```python
from build123d import *

# Parameters (mm, degrees)
PAD_DEPTH       = 20
SKETCH001_R     = 4.5
POCKET_DEPTH    = 107.001
SKETCH002_R     = 8.25
POCKET001_DEPTH = 25
POCKET002_DEPTH = 10
SKETCH004_R     = 1.5
POCKET003_DEPTH = 10.001
SKETCH005_R     = 5.5
POCKET004_DEPTH = 10
SKETCH006_W     = 23
SKETCH006_H     = 12
POCKET005_DEPTH = 3
SKETCH007_R     = 1.5
POCKET006_DEPTH = 7.001


with BuildPart() as part:
    # Sketch → Pad (new body)
    with BuildSketch(Plane.XY):
        with BuildLine():
            ThreePointArc((0, 57.5), (-57.5, 0), (0, -57.5))
            Line((0, -57.5), (0, -93.245553))
            Line((0, -93.245553), (-30, -93.245553))
            Line((-30, -93.245553), (-30, -63.245553))
            ThreePointArc((-55.235858, -43), (-43.803635, -54.600747), (-30, -63.245553))
            Line((-107, -20), (-55.235858, -43))
            Line((-107, 20), (-107, -20))
            Line((-55.235858, 43), (-107, 20))
            ThreePointArc((-30, 63.245553), (-43.803635, 54.600747), (-55.235858, 43))
            Line((-30, 93.245553), (-30, 63.245553))
            Line((0, 93.245553), (-30, 93.245553))
            Line((0, 57.5), (0, 93.245553))
        make_face()
        with BuildLine():
            Line((-63.245553, 30), (-97, 15))
            Line((-97, 15), (-97, -15))
            Line((-97, -15), (-63.245553, -30))
            ThreePointArc((-63.245553, 30), (-70, 0), (-63.245553, -30))
        make_face(mode=Mode.SUBTRACT)
    extrude(amount=PAD_DEPTH)

    # Sketch001 (on Face2 of Pad) → Pocket (cut, through all)
    with BuildSketch(Plane.YZ):
        with Locations((-78.25, 10)):
            Circle(SKETCH001_R)
        with Locations((78.25, 10)):
            Circle(SKETCH001_R)
    extrude(amount=-POCKET_DEPTH, mode=Mode.SUBTRACT)

    # Sketch002 (on Face3 of Pocket) → Pocket001 (cut)
    with BuildSketch(Plane.YZ.offset(-2.5)):
        with Locations((-78.25, 10)):
            Circle(SKETCH002_R)
        with Locations((78.25, 10)):
            Circle(SKETCH002_R)
    extrude(amount=-POCKET001_DEPTH, mode=Mode.SUBTRACT)

    # Sketch003 (on Face5 of Pocket001) → Pocket002 (cut)
    with BuildSketch(Plane.XY.offset(20)):
        with BuildLine():
            ThreePointArc((0, 70), (-16.341175, 68.065894), (-31.779335, 62.370457))
            Line((-31.779335, 62.370457), (-31.779335, 95))
            Line((-31.779335, 95), (0, 95))
            Line((0, 95), (0, 70))
        make_face()
        with BuildLine():
            ThreePointArc((-31.779335, -62.370457), (-16.341175, -68.065894), (0, -70))
            Line((0, -95), (0, -70))
            Line((-31.779335, -95), (0, -95))
            Line((-31.779335, -62.370457), (-31.779335, -95))
        make_face()
    extrude(amount=-POCKET002_DEPTH, mode=Mode.SUBTRACT)

    # Sketch004 (on Face11 of Pocket002) → Pocket003 (cut, through all)
    with BuildSketch(Plane.XY.offset(10)):
        with Locations((-22.5, 90.25)):
            Circle(SKETCH004_R)
        with Locations((-7.5, 90.25)):
            Circle(SKETCH004_R)
        with Locations((-7.5, -90.25)):
            Circle(SKETCH004_R)
        with Locations((-22.5, -90.25)):
            Circle(SKETCH004_R)
    extrude(amount=-POCKET003_DEPTH, mode=Mode.SUBTRACT)

    # Sketch005 (on Face20 of Pocket003) → Pocket004 (cut)
    with BuildSketch(Plane(origin=(-107, 0, 0), x_dir=(0, -1, 0), z_dir=(-1, 0, 0))):
        with Locations((0, 10)):
            Circle(SKETCH005_R)
    extrude(amount=-POCKET004_DEPTH, mode=Mode.SUBTRACT)

    # Sketch006 (on Face25 of Pocket004) → Pocket005 (cut)
    with BuildSketch(Plane.YZ.offset(-97)):
        with Locations((0, 10)):
            Rectangle(SKETCH006_W, SKETCH006_H)
    extrude(amount=-POCKET005_DEPTH, mode=Mode.SUBTRACT)

    # Sketch007 (on Face42 of Pocket005) → Pocket006 (cut, through all)
    with BuildSketch(Plane.YZ.offset(-100)):
        with Locations((-8, 10)):
            Circle(SKETCH007_R)
        with Locations((8, 10)):
            Circle(SKETCH007_R)
    extrude(amount=-POCKET006_DEPTH, mode=Mode.SUBTRACT)


solid = part.part
```
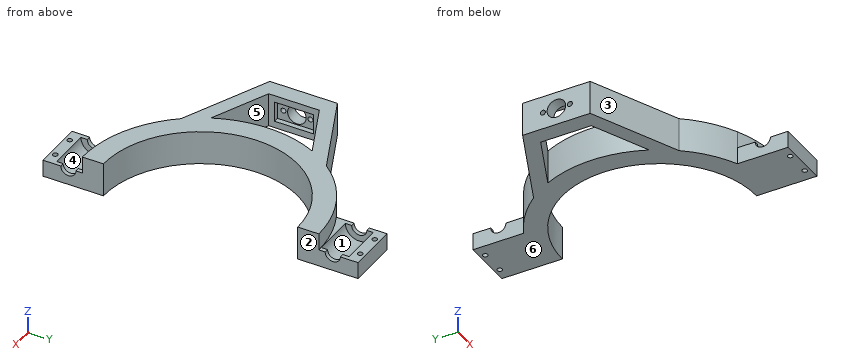
Geometry check sheet. Reference: the model listing, model coordinates, mm. Face numbers are marked on the shaded views. A direction names the side the tool comes from. Coordinates: 2 decimals unless noted, no trailing zeros. Order: outer loops, then holes, each group sorted by start corner. A loop starts at its lowest first (then second) coordinate and runs counter-clockwise, first axis right, second up. Notation, with made-up numbers: (-32.5, 87.25) - (-4.5, 87.25) arc R13 cw to (-4.5, 92.25) - close; hole circle Ø9 at (-20.75, 45.5). An arc over 180 degrees is marked (long way). Answer as a JSON object with one key per item and string values. Group by question number.
Item 1: Sectioned sample at B-B, the plane x = -12. Record the cut outline in (y, z).
Item 2: Sectioned sample at D-D, the plane x = -89. Record the cut outline in (y, z), and give its area (3 significant figures).
Item 3: Tool access check on the marked faces 4, 5 and 6. Record the directions out of +Z, -Z, +X, -X, +Y, -Y that give a thin tool (end or side, any length) a straight path to the whole face; none if there is none.
Item 4: Scan lines: probe 1 along X at (y, z) = (90.25, 5.25); probe 2 along X at (y, z) = (-82, 3.25); probe 3 along Y at (x, z) = (-7.5, 2.75). Record each from-to range of solid material in increasing order.
Item 5: Sectioned sample at C-C, the plane y = -78.5. Record the cut outline in (x, z), and give its area (3 significant figures).
Item 6: Sectioned sample at A-A, the plane y = 0. Record the cut outline in (x, z), and give its area (3 significant figures).
Item 7: Draft check along Y on the marked faces 1, 2 and 3. Enter one of: +Y half, -Y half, draft (parallel to the pull), parting line (faces both ways), or undercut.
Item 8: Depth check by flat-ended pin: pin 1 Ø10 at (y, z) = (7.5, 5.5) entering from +X; pin 2 Ø11 at (y, z) = (74.5, 3.5) entering from -X; pin 3 Ø10 at (x, z) = (-36.5, 6) entering from +Y; pin 4 Ø1.8 at (x, y) = (-7.5, 90.25) entering from -Z. Enter the tip coordinate at first touch or a pass-through.
Resolved:
{
 "1": {"outline": "(-93.25, 0) - (-56.23, 0) - (-56.23, 20) - (-68.96, 20) - (-68.96, 10) - (-70, 10) arc R8.25 cw to (-86.5, 10) - (-93.25, 10) - close; (56.23, 0) - (93.25, 0) - (93.25, 10) - (86.5, 10) arc R8.25 cw to (70, 10) - (68.96, 10) - (68.96, 20) - (56.23, 20) - close"},
 "2": {"outline": "(-28, 0) - (-18.56, 0) - (-18.56, 20) - (-28, 20) - close; (18.56, 0) - (28, 0) - (28, 20) - (18.56, 20) - close", "area": "378 mm^2"},
 "3": {"face 4": "+Z", "face 5": "+Z, -Z", "face 6": "-Z, +X, -X, +Y, -Y"},
 "4": {"probe 1": "-30 to -24, -21 to -9, -6 to 0", "probe 2": "-30 to -27.5, -2.5 to 0", "probe 3": "-93.25 to -91.75, -88.75 to -82.19, -74.31 to -57.01, 57.01 to 74.31, 82.19 to 88.75, 91.75 to 93.25"},
 "5": {"outline": "(-30, 0) - (0, 0) - (0, 5.51) - (-2.5, 5.51) - (-2.5, 1.75) - (-27.5, 1.75) - (-27.5, 5.51) - (-30, 5.51) - close", "area": "71.4 mm^2"},
 "6": {"outline": "(-107, 0) - (-97, 0) - (-97, 4) - (-100, 4) - (-100, 4.5) - (-107, 4.5) - close; (-107, 15.5) - (-100, 15.5) - (-100, 16) - (-97, 16) - (-97, 20) - (-107, 20) - close; (-70, 0) - (-57.5, 0) - (-57.5, 20) - (-70, 20) - close", "area": "337 mm^2"},
 "7": {"face 1": "undercut", "face 2": "draft", "face 3": "-Y half"},
 "8": {"pin 1": "x = -56.12", "pin 2": "x = -30", "pin 3": "y = 62.51", "pin 4": "through"}
}
